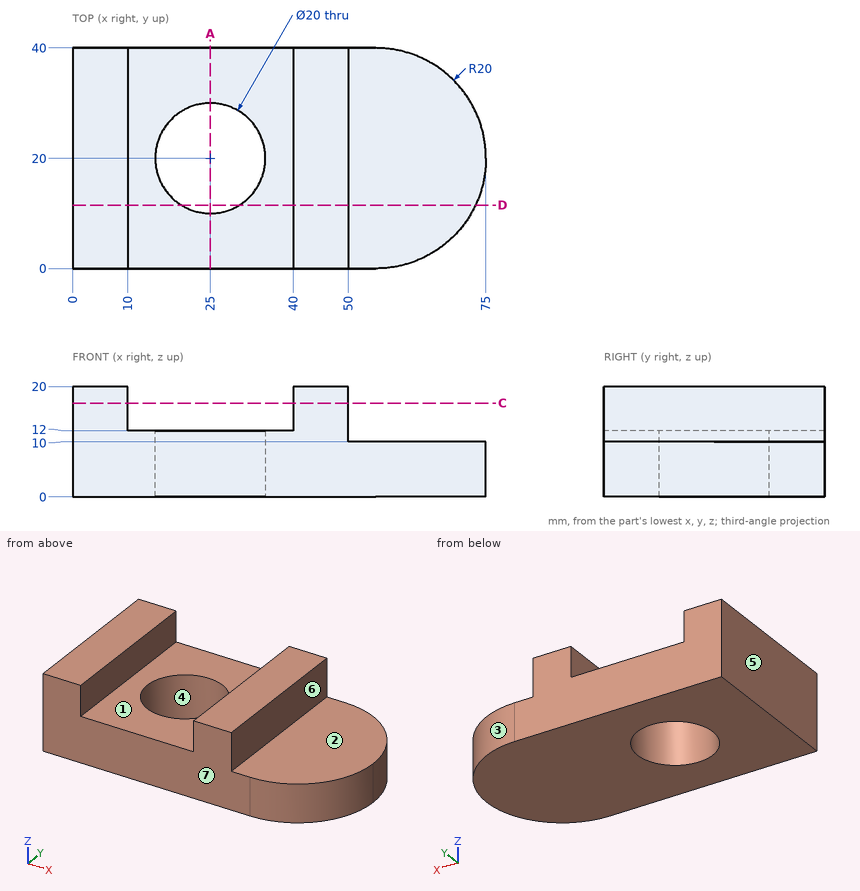
Drawing for the job (mm, zero at the part's lowest x, y, z). A direction names the side the tool comes from. Coordinates: 2 decimals unless noted, no trailing zeros. Loops run counter-clockwise (first coordinate to the right, second up) from the corner with the lowest first, then second, coordinate; pieces in that order, holes last. Notation, with made-up numbers: (50.5, -17) - (106.5, -17) arc R20 ccw to (106.5, 1) - close; hole circle Ø11 at (52.5, 7). An arc over 180 degrees is marked (long way). Use CSV: the item, a comma, the result in double quotes. Start each with the question number.
Q1. Probe probe 1 along X at (y, z) = (33, 18); probe 2 along Y at (x, z) = (25, 6.5); probe 3 along Z at (x, y) = (30, 4). List the from-to ranges inside material, lowest first. Write a range as from..to.
Q2. Cut at C-C, the plane z = 17. List the corners of the cut face in (x, y), then the cut area to 3 significant figures.
Q3. 3-axis set-ups, long thin cutter, end or side, ignore diameter. For the marked faces 1, 2 and 3: which of +Z, -Z, +X, -X, +Y, -Y reach the whole face in a straight line?
Q4. Cut at A-A, the plane x = 25. List the corners of the cut face in (y, z).
Q5. Cut at D-D, the plane y = 11.5. List the corners of the cut face in (x, z).
Q6. Drop flat-ended pins along their axis: P1, Ø1, axis at y = 12, z = 3.5, coming from the +X side; P2, Ø4, axis at x = 37.5, y = 21.5, coming from the +Z side; P3, Ø8, axis at y = 23.5, z = 15.5, coming from the +X side. Give the stop position or say it passes through.
Q7. Two-plate mould, pull along X, no slides. Class the marked faces 4, 5, 6 and 7: +X half, -X half, draft (parallel to the pull), parting line (faces both ways), or undercut.
Here are the results:
1,probe 1,"0..10, 40..50"
1,probe 2,"0..10, 30..40"
1,probe 3,"0..12"
2,outline,"(0, 0) - (10, 0) - (10, 40) - (0, 40) - close; (40, 0) - (50, 0) - (50, 40) - (40, 40) - close"
2,area,"800 mm2"
3,face 1,"+Z, +Y, -Y"
3,face 2,"+Z, +X, +Y, -Y"
3,face 3,"+Z, -Z, +X, +Y"
4,outline,"(0, 0) - (10, 0) - (10, 12) - (0, 12) - close; (30, 0) - (40, 0) - (40, 12) - (30, 12) - close"
5,outline,"(0, 0) - (19.73, 0) - (19.73, 12) - (10, 12) - (10, 20) - (0, 20) - close; (30.27, 0) - (73.1, 0) - (73.1, 10) - (50, 10) - (50, 20) - (40, 20) - (40, 12) - (30.27, 12) - close"
6,P1,"x = 73.54"
6,P2,"z = 12"
6,P3,"x = 50"
7,face 4,"undercut"
7,face 5,"-X half"
7,face 6,"+X half"
7,face 7,"draft"
